from build123d import *

# Parameters (mm, degrees)
BOSS_EXTRUDE1_DEPTH     = 14.224
CUT_EXTRUDE1_DEPTH      = 11.684
FILLET1_R               = 2.54
SKETCH3_W               = 32.258
SKETCH3_H               = 8.128
CUT_EXTRUDE2_DEPTH      = 1
CUT_EXTRUDE2_DEPTH_BACK = 48.498
SKETCH5_W               = 26.924
SKETCH5_H               = 34.29
CUT_EXTRUDE4_DEPTH      = 1.524
SKETCH6_W               = 20.290608306
SKETCH6_H               = 27.072145664
CUT_EXTRUDE5_DEPTH      = 1.524
BOSS_EXTRUDE2_DEPTH     = 0.762
SKETCH8_W               = 12.7
SKETCH8_H               = 0.762
BOSS_EXTRUDE3_DEPTH     = 4.064


with BuildPart() as part:
    # Sketch1 → Boss-Extrude1 (new body)
    with BuildSketch(Plane.XY):
        with BuildLine():
            Line((-21.209, -23.749), (21.209, -23.749))
            ThreePointArc((21.209, -23.749), (23.005051224, -23.005051224), (23.749, -21.209))
            Line((23.749, -21.209), (23.749, 21.209))
            ThreePointArc((23.749, 21.209), (23.005051224, 23.005051224), (21.209, 23.749))
            Line((21.209, 23.749), (-21.209, 23.749))
            ThreePointArc((-21.209, 23.749), (-23.005051224, 23.005051224), (-23.749, 21.209))
            Line((-23.749, 21.209), (-23.749, -21.209))
            ThreePointArc((-23.749, -21.209), (-23.005051224, -23.005051224), (-21.209, -23.749))
        make_face()
    extrude(amount=BOSS_EXTRUDE1_DEPTH)

    # Sketch2 → Cut-Extrude1 (cut)
    with BuildSketch(Plane.XY.offset(14.224)):
        with BuildLine():
            Line((19.939, -22.479), (-19.939, -22.479))
            ThreePointArc((-19.939, -22.479), (-21.735051224, -21.735051224), (-22.479, -19.939))
            Line((-22.479, -19.939), (-22.479, 19.939))
            ThreePointArc((-22.479, 19.939), (-21.735051224, 21.735051224), (-19.939, 22.479))
            Line((-19.939, 22.479), (19.939, 22.479))
            ThreePointArc((19.939, 22.479), (21.735051224, 21.735051224), (22.479, 19.939))
            Line((22.479, 19.939), (22.479, -19.939))
            ThreePointArc((22.479, -19.939), (21.735051224, -21.735051224), (19.939, -22.479))
        make_face()
    extrude(amount=-CUT_EXTRUDE1_DEPTH, mode=Mode.SUBTRACT)

    # Fillet1
    fillet1_edges = [part.edges().sort_by_distance(p)[0] for p in [
        (0, -23.749, 0),
        (-23.005051224, -23.005051224, 0),
        (-23.749, 0, 0),
        (-23.005051224, 23.005051224, 0),
        (0, 23.749, 0),
        (23.005051224, 23.005051224, 0),
        (23.749, 0, 0),
        (23.005051224, -23.005051224, 0),
    ]]
    fillet(fillet1_edges, radius=FILLET1_R)

    # Sketch3 → Cut-Extrude2 (cut, two sides)
    with BuildSketch(Plane(origin=(0, 23.749, 0), x_dir=(1, 0, 0), z_dir=(0, 1, 0))) as cut_extrude2_sk:
        with Locations((0, -14.224)):
            Rectangle(SKETCH3_W, SKETCH3_H)
    extrude(amount=CUT_EXTRUDE2_DEPTH, mode=Mode.SUBTRACT)
    extrude(cut_extrude2_sk.sketch, amount=-CUT_EXTRUDE2_DEPTH_BACK, mode=Mode.SUBTRACT)

    # Sketch5 → Cut-Extrude4 (cut)
    with BuildSketch(Plane(origin=(0, 0, 0), x_dir=(-1, 0, 0), z_dir=(0, 0, -1))):
        Rectangle(SKETCH5_W, SKETCH5_H)
    extrude(amount=-CUT_EXTRUDE4_DEPTH, mode=Mode.SUBTRACT)

    # Sketch6 → Cut-Extrude5 (cut)
    with BuildSketch(Plane(origin=(0, 0, 1.524), x_dir=(-1, 0, 0), z_dir=(0, 0, -1))):
        Rectangle(SKETCH6_W, SKETCH6_H)
    extrude(amount=-CUT_EXTRUDE5_DEPTH, mode=Mode.SUBTRACT)

    # Sketch7 → Boss-Extrude2 (add)
    with BuildSketch(Plane(origin=(0, 0, 0), x_dir=(-1, 0, 0), z_dir=(0, 0, -1))):
        with BuildLine():
            Line((19.939, 17.145), (21.209, 17.145))
            ThreePointArc((21.209, 17.145), (17.399, 20.955), (13.589, 17.145))
            Line((13.589, 17.145), (14.859, 17.145))
            ThreePointArc((14.859, 17.145), (17.399, 19.685), (19.939, 17.145))
        make_face()
        with BuildLine():
            Line((21.209, 15.875), (16.129, 15.875))
            ThreePointArc((16.129, 15.875), (13.589, 13.335), (16.129, 10.795))
            Line((16.129, 10.795), (21.209, 10.795))
            Line((21.209, 10.795), (21.209, 12.065))
            Line((21.209, 12.065), (16.129, 12.065))
            ThreePointArc((16.129, 12.065), (14.859, 13.335), (16.129, 14.605))
            Line((16.129, 14.605), (21.209, 14.605))
            Line((21.209, 14.605), (21.209, 15.875))
        make_face()
        Polygon((13.589, 9.525), (21.209, 9.525), (21.209, 5.715), (19.939, 5.715), (19.939, 8.255), (18.034, 8.255), (18.034, 6.985), (16.764, 6.985), (16.764, 8.255), (13.589, 8.255), align=None)
        Polygon((13.589, 4.445), (21.209, 4.445), (21.209, 0.635), (19.939, 0.635), (19.939, 3.175), (18.034, 3.175), (18.034, 1.905), (16.764, 1.905), (16.764, 3.175), (13.589, 3.175), align=None)
        Polygon((21.209, -0.635), (13.589, -0.635), (13.589, -4.445), (14.859, -4.445), (14.859, -1.905), (21.209, -1.905), align=None)
        Polygon((13.589, -5.715), (21.209, -5.715), (21.209, -9.525), (19.939, -9.525), (19.939, -6.985), (18.034, -6.985), (18.034, -8.255), (16.764, -8.255), (16.764, -6.985), (14.859, -6.985), (14.859, -9.525), (13.589, -9.525), align=None)
        with BuildLine():
            Line((18.9865, -13.97), (18.9865, -15.24))
            ThreePointArc((18.9865, -15.24), (20.558044821, -11.445955179), (16.764, -13.0175))
            ThreePointArc((16.764, -13.0175), (15.137980791, -13.691019209), (15.8115, -12.065))
            Line((15.8115, -12.065), (15.8115, -10.795))
            ThreePointArc((15.8115, -10.795), (14.239955179, -14.589044821), (18.034, -13.0175))
            ThreePointArc((18.034, -13.0175), (19.660019209, -12.343980791), (18.9865, -13.97))
        make_face()
        with BuildLine():
            Line((15.8115, -17.78), (15.8115, -16.51))
            ThreePointArc((15.8115, -16.51), (14.239955179, -20.304044821), (18.034, -18.7325))
            ThreePointArc((18.034, -18.7325), (19.660019209, -18.058980791), (18.9865, -19.685))
            Line((18.9865, -19.685), (18.9865, -20.955))
            ThreePointArc((18.9865, -20.955), (20.558044821, -17.160955179), (16.764, -18.7325))
            ThreePointArc((16.764, -18.7325), (15.137980791, -19.406019209), (15.8115, -17.78))
        make_face()
    extrude(amount=BOSS_EXTRUDE2_DEPTH)

    # Sketch8 → Boss-Extrude3 (add)
    with BuildSketch(Plane.XY.offset(10.16)):
        with Locations((0, 22.86)):
            Rectangle(SKETCH8_W, SKETCH8_H)
        with Locations((0, -22.86)):
            Rectangle(SKETCH8_W, SKETCH8_H)
    extrude(amount=BOSS_EXTRUDE3_DEPTH)


solid = part.part
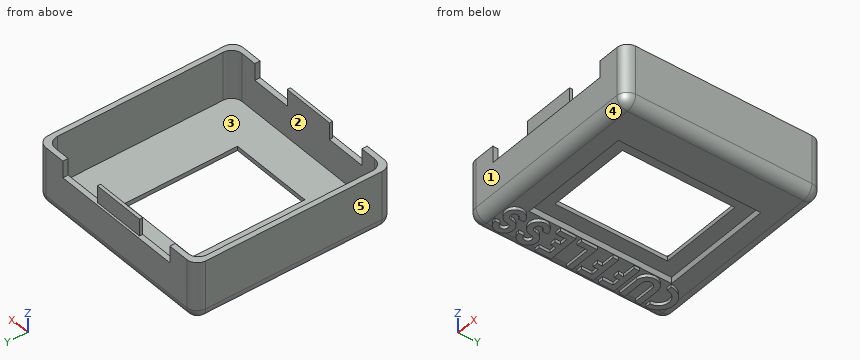
Can you work these out from the model? Positions are in its coordinate system, mm. Face numbers are marked on the shaded views. A direction names the side the tool comes from. Round coordinates to 2 decimals unless told otherwise and drop trailing zeros. Loops run counter-clockwise (first coordinate to the right, second up) from the corner with the lowest first, then second, coordinate; pieces in that order, holes last. Notation, with made-up numbers: (37.5, 49.25) - (64.5, 49.25) arc R13 ccw to (64.5, 53.25) - close; hole circle Ø3 at (-17.75, -20). An arc over 180 degrees is marked (long way). Answer in a Markdown table with one row per item. Add a question column.
Q1. I want a section at D-D on z = 6. List the corners of the cut face in (x, y) for me.
Q2. Which directions (+Z, -Z, +X, -X, +Y, -Y) give clear straight access to the entire face, cutting with the end or side of a thin tool? Please do the marked faces 1 and 2.
Q3. We'd pull the mould along X, two halves only. Please class the marked faces 3, 4 and 5: pulls with the +X half, pulls with the -X half, needs draft (parallel to the pull), parting line crosses it, or undercut.
Q4. I want a section at A-A on x = 3. List the corners of the cut face in (y, z) for me (3 decimals), and give its area (3 significant figures).
Q5. I need wall thicknesses on L1, parallel to X at y = -18.5, z = 5.25; L2, parallel to Z at x = 13, y = -10. Which ranges of each line are inside material? Lowest first, please.
Q6. I want a section at B-B on z = 12.5. Count the separate pieces of the cut face and the enclosed holes in it, and give its area (3 significant figures).
Q7. I want a section at C-C on y = -2.5. List the corners of the cut face in (x, z) for me, and give its area (3 significant figures).
Q8. For pin 1 Ø0.5 at (y, z) = (1.5, 2) entering from +X; pin 2 Ø0.5 at (y, z) = (-8.5, 1) entering from -X; pin 3 Ø10 at (x, y) = (-13, 6.5) entering from +Z; pin 4 Ø8 at (x, y) = (4, 7.5) entering from -Z, each with a flat end and sliding along its axis, tell me the tip position at first contact or that it passes through.
A:
| question | item | result |
|---|---|---|
| 1 | outline | (-23.75, -21.21) arc R2.54 ccw to (-21.21, -23.75) - (21.21, -23.75) arc R2.54 ccw to (23.75, -21.21) - (23.75, 21.21) arc R2.54 ccw to (21.21, 23.75) - (-21.21, 23.75) arc R2.54 ccw to (-23.75, 21.21) - close; hole (-22.48, -19.94) arc R2.54 ccw to (-19.94, -22.48) - (19.94, -22.48) arc R2.54 ccw to (22.48, -19.94) - (22.48, 19.94) arc R2.54 ccw to (19.94, 22.48) - (-19.94, 22.48) arc R2.54 ccw to (-22.48, 19.94) - close |
| 2 | face 1 | +Z, -Z, +X, -X, -Y |
| 2 | face 2 | +Z |
| 3 | face 3 | undercut |
| 3 | face 4 | needs draft |
| 3 | face 5 | pulls with the -X half |
| 4 | outline | (-23.749, 2.54) arc R2.54 ccw to (-21.209, 0) - (-17.145, 0) - (-17.145, 1.524) - (-13.536, 1.524) - (-13.536, 2.54) - (-22.479, 2.54) - (-22.479, 14.224) - (-23.241, 14.224) - (-23.241, 10.16) - (-23.749, 10.16) - close; (13.536, 1.524) - (17.145, 1.524) - (17.145, 0) - (21.209, 0) arc R2.54 ccw to (23.749, 2.54) - (23.749, 10.16) - (23.241, 10.16) - (23.241, 14.224) - (22.479, 14.224) - (22.479, 2.54) - (13.536, 2.54) - close |
| 4 | area | 63.7 mm^2 |
| 5 | L1 | -23.75 to -22.48, 22.48 to 23.75 |
| 5 | L2 | 1.52 to 2.54 |
| 6 | separate pieces | 4 |
| 6 | enclosed holes | 0 |
| 6 | area | 172 mm^2 |
| 7 | outline | (-23.75, 2.54) arc R2.54 ccw to (-21.21, 0) - (-14.86, 0) - (-14.86, -0.76) - (-13.59, -0.76) - (-13.59, 0) - (-13.46, 0) - (-13.46, 1.52) - (-10.15, 1.52) - (-10.15, 2.54) - (-22.48, 2.54) - (-22.48, 14.22) - (-23.75, 14.22) - close; (10.15, 1.52) - (13.46, 1.52) - (13.46, 0) - (21.21, 0) arc R2.54 ccw to (23.75, 2.54) - (23.75, 14.22) - (22.48, 14.22) - (22.48, 2.54) - (10.15, 2.54) - close |
| 7 | area | 86.9 mm^2 |
| 8 | pin 1 | x = 23.73 |
| 8 | pin 2 | x = -23.4 |
| 8 | pin 3 | z = 2.54 |
| 8 | pin 4 | through |
